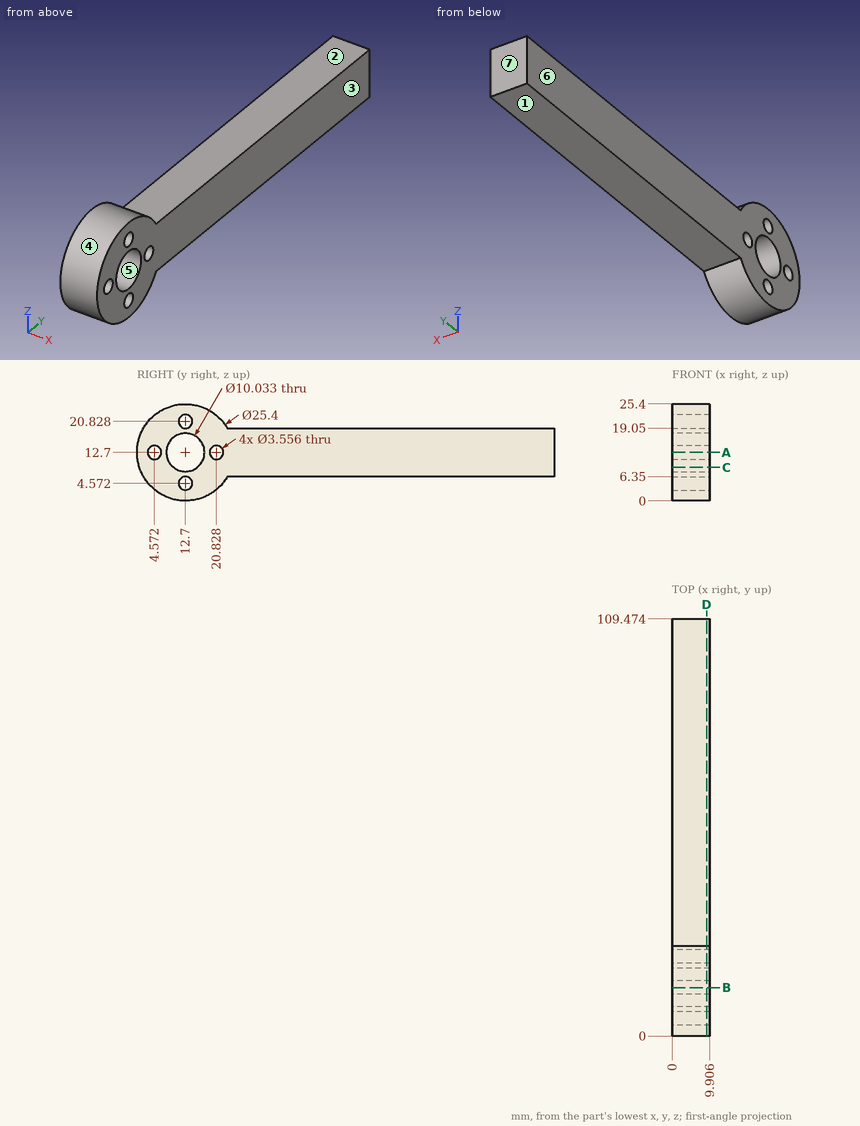
The drawing under review shows one solid part. Ordinate dimensions are in mm from its lowest x, y, z. A direction names the side the tool comes from. Coordinates: 2 decimals unless noted, no trailing zeros. Order: outer loops, then holes, each group sorted by start corner. A loop starts at its lowest first (then second) coordinate and runs counter-clockwise, first axis right, second up. Notation, with made-up numbers: (69, 10) -> (90, 10) arc R20 cw to (90, 37) -> close; hole circle Ø9 at (27, 14.5). An arc over 180 degrees is marked (long way). Answer in a Markdown table with one row per item.
(1) Consider section B-B (y = 12.7). Write out the cut boundary in (x, z).
Answers:
| item | result |
|---|---|
| outline | (0, 0) -> (9.91, 0) -> (9.91, 2.79) -> (0, 2.79) -> close; (0, 6.35) -> (9.91, 6.35) -> (9.91, 7.68) -> (0, 7.68) -> close; (0, 17.72) -> (9.91, 17.72) -> (9.91, 19.05) -> (0, 19.05) -> close; (0, 22.61) -> (9.91, 22.61) -> (9.91, 25.4) -> (0, 25.4) -> close |
(2) Insertion check: pin 1 (5 mm diameter, centred on x = 4.5, y = 49.5, fed in from -Z); pin 2 (5 mm diameter, centred on x = 5, z = 16.5, fed in from -Y); pin 3 (3 mm diameter, centred on x = 7, z = 21, fed in from -Y). Each pin has a flat end and moves straight along its axis. Give the tip position at first contact, or say it passes through.
Answers:
| item | result |
|---|---|
| pin 1 | z = 6.35 |
| pin 2 | y = 0.07 |
| pin 3 | y = 1.97 |
(3) The part is to be moulded in two halves that separate along Y. For the marked faces 4, 5, 6 and 7, say which applies: +Y half, -Y half, draft (parallel to the pull), parting line (faces both ways), or undercut.
Answers:
| item | result |
|---|---|
| face 4 | parting line |
| face 5 | undercut |
| face 6 | draft |
| face 7 | +Y half |
(4) Machinability: for the marked faces 1, 2 and 3, which of the approach directions +Z, -Z, +X, -X, +Y, -Y give a long, thin tool a straight path to every point of the face, cutting with its end or side? Answer none if there is none.
Answers:
| item | result |
|---|---|
| face 1 | -Z, +X, -X, +Y |
| face 2 | +Z, +X, -X, +Y |
| face 3 | +Z, -Z, +X, +Y, -Y |
(5) Consider section C-C (z = 8.75). Write out the cut boundary in (x, y).
Answers:
| item | result |
|---|---|
| outline | (0, 0.63) -> (9.91, 0.63) -> (9.91, 9.61) -> (0, 9.61) -> close; (0, 15.79) -> (9.91, 15.79) -> (9.91, 109.47) -> (0, 109.47) -> close |
(6) Consider section A-A (z = 12.7). Write out the cut boundary in (x, y).
Answers:
| item | result |
|---|---|
| outline | (0, 0) -> (9.91, 0) -> (9.91, 2.79) -> (0, 2.79) -> close; (0, 6.35) -> (9.91, 6.35) -> (9.91, 7.68) -> (0, 7.68) -> close; (0, 17.72) -> (9.91, 17.72) -> (9.91, 19.05) -> (0, 19.05) -> close; (0, 22.61) -> (9.91, 22.61) -> (9.91, 109.47) -> (0, 109.47) -> close |
(7) Consider section D-D (x = 9). Write out the cut boundary in (y, z).
Answers:
| item | result |
|---|---|
| outline | (23.7, 6.35) -> (109.47, 6.35) -> (109.47, 19.05) -> (23.7, 19.05) arc R12.7 ccw (long way) to start; hole circle Ø3.56 at (4.57, 12.7); hole circle Ø10.03 at (12.7, 12.7); hole circle Ø3.56 at (12.7, 4.57); hole circle Ø3.56 at (12.7, 20.83); hole circle Ø3.56 at (20.83, 12.7) |
(8) Wall thickness on line 1 along Y through (x, z) = (6.5, 12.7); line 2 along Y through (x, z) = (8.5, 13.25); line 3 along Z through (x, y) = (4.5, 40.5): over which ranges is each line inside the solid? List them lowest first.
Answers:
| item | result |
|---|---|
| line 1 | 0 to 2.79, 6.35 to 7.68, 17.72 to 19.05, 22.61 to 109.47 |
| line 2 | 0.01 to 2.88, 6.26 to 7.71, 17.69 to 19.14, 22.52 to 109.47 |
| line 3 | 6.35 to 19.05 |
